Design review of the part built by this model. Coordinates are the model's own, in mm. A direction names the side the tool comes from. Coordinates: 2 decimals unless noted, no trailing zeros. Loops run counter-clockwise (first coordinate to the right, second up) from the corner with the lowest first, then second, coordinate; pieces in that order, holes last.
Q1. Add section D-D on x = 88.5. Give the boundary of the cut face in (y, z).
Q2. Draft analysis for pull direction Z (two halves, no side actions). For faces 1 (the face through (61, 51.9, 149.3)), 2 (the face through (60, 50, 0)), 3 (the face through (42.73, 51.78, 67.63)), 4 (the face through (0, 22, 54)), state which applies: released by +Z, released by -Z, zero draft, split by the parting line, or undercut.
Q3. Machinability: for faces 5 (the face through (-3.13, 4.51, 105.72)), 6 (the face through (81.41, 51.87, 74.04)), which of the approach directions +Z, -Z, +X, -X, +Y, -Y give a long, thin tool a straight path to every point of the face, cutting with its end or side? Answer none if there is none.
Q4. Add section A-A on z = 36.5. Give the boundary of the cut face in (x, y), and give its area (3 significant figures).
Q5. For P1, Ø3, axis at x = 60.5, y = 50.5, coming from the +Z side; P2, Ø3, axis at y = 52.5, z = 41.5, coming from the +X side; P3, Ø7, axis at y = 51, z = 54.5, coming from the +X side; P4, Ø1.1, axis at x = 47, y = 51, coming from the -Z side, all flat-tipped, find the tip position at first contact; note any pin that passes through.
Q6. Add section C-C on y = 21. Give the boundary of the cut face in (x, z).
Q7. Wall thickness on probe 1 along X at (y, z) = (24.5, 41); probe 2 along Y at (x, z) = (69.5, 23.5); probe 3 along X at (y, z) = (51, 26): over which ranges is each line inside the solid? List them lowest first.
Q8. Add section B-B on y = 43.5. Give the boundary of the cut face in (x, z).
```python
from build123d import *

# Parameters (mm, degrees)
BRIDA_BASE1_DEPTH          = 110
PESTA_A1_DEPTH             = 6.35
CORTAR_EXTRUIR1_REACH      = 205.181
REDONDEO1_R                = 15
CORTAR_EXTRUIR3_DEPTH      = 204.181381454
CORTAR_EXTRUIR3_DEPTH_BACK = 204.181381454
CROQUIS11_R                = 5.125
REDONDEO2_R                = 2
REDONDEO3_R                = 5


# Sheet-metal steps are written as plain solids
with BuildPart() as part:
    # Croquis1 → Brida base1 (new body)
    with BuildSketch(Plane.XY):
        with BuildLine():
            Line((0, 0), (0, 45.47))
            ThreePointArc((0, 45.47), (0.931400436, 47.718599564), (3.18, 48.65))
            Line((3.18, 48.65), (116.82, 48.65))
            ThreePointArc((116.82, 48.65), (119.068599564, 47.718599564), (120, 45.47))
            Line((120, 45.47), (120, 0))
            Line((120, 0), (126.35, 0))
            Line((126.35, 0), (126.35, 45.47))
            ThreePointArc((126.35, 45.47), (123.558727625, 52.208727625), (116.82, 55))
            Line((116.82, 55), (3.18, 55))
            ThreePointArc((3.18, 55), (-3.558727625, 52.208727625), (-6.35, 45.47))
            Line((-6.35, 45.47), (-6.35, 0))
            Line((-6.35, 0), (0, 0))
        make_face()
    extrude(amount=BRIDA_BASE1_DEPTH)

    # Croquis6 → Pestaña1 (add)
    with BuildSketch(Plane(origin=(0, 55, 0), x_dir=(1, 0, 0), z_dir=(0, 1, 0))):
        with BuildLine():
            Line((3.18, -110), (116.82, -110))
            ThreePointArc((116.82, -110), (60, -149.309581975), (3.18, -110))
        make_face()
    extrude(amount=-PESTA_A1_DEPTH)

    # Croquis9 → Cortar-Extruir1 (cut, up to next)
    with BuildSketch(Plane(origin=(0, 55, 0), x_dir=(1, 0, 0), z_dir=(0, 1, 0)), mode=Mode.PRIVATE) as cortar_extruir1_sk1:
        with BuildLine():
            Line((53.25, -115), (85.45, -115))
            Line((85.45, -115), (85.45, -93))
            ThreePointArc((85.45, -93), (79.1, -86.65), (72.75, -93))
            Line((72.75, -93), (66.75, -101))
            Line((66.75, -101), (66.75, -78))
            Line((66.75, -78), (77.45, -78))
            Line((77.45, -78), (85.45, -70))
            Line((85.45, -70), (85.45, -58))
            ThreePointArc((85.45, -58), (79.1, -51.65), (72.75, -58))
            Line((72.75, -58), (66.75, -66))
            Line((66.75, -66), (66.75, -25))
            Line((66.75, -25), (53.25, -25))
            Line((53.25, -25), (53.25, -56))
            Line((53.25, -56), (47.25, -48))
            ThreePointArc((47.25, -48), (40.9, -41.65), (34.55, -48))
            Line((34.55, -48), (34.55, -60))
            Line((34.55, -60), (42.55, -68))
            Line((42.55, -68), (53.25, -68))
            Line((53.25, -68), (53.25, -91))
            Line((53.25, -91), (47.25, -83))
            ThreePointArc((47.25, -83), (40.9, -76.65), (34.55, -83))
            Line((34.55, -83), (34.55, -105))
            Line((34.55, -105), (53.25, -105))
            Line((53.25, -105), (53.25, -115))
        make_face()
    cortar_extruir1_tool1 = extrude(cortar_extruir1_sk1.sketch, amount=-CORTAR_EXTRUIR1_REACH, mode=Mode.PRIVATE) & part.part
    add(cortar_extruir1_tool1.solids().sort_by_distance((60, 55, 76.162835))[0], mode=Mode.SUBTRACT)

    # Redondeo1
    redondeo1_edges = [part.edges().sort_by_distance(p)[0] for p in [
        (-3.175, 0, 0),
        (123.175, 0, 0),
        (-3.175, 0, 110),
        (123.175, 0, 110),
    ]]
    fillet(redondeo1_edges, radius=REDONDEO1_R)

    # Croquis11 → Cortar-Extruir3 (cut, two sides: drawn at the far end of the back side and taken through both)
    with BuildSketch(Plane.ZY.offset(-120).offset(-CORTAR_EXTRUIR3_DEPTH_BACK)):
        with Locations((20.003172622, 22.868986368)):
            Circle(CROQUIS11_R)
        with Locations((90.003172622, 22.868986368)):
            Circle(CROQUIS11_R)
    extrude(amount=CORTAR_EXTRUIR3_DEPTH + CORTAR_EXTRUIR3_DEPTH_BACK, mode=Mode.SUBTRACT)

    # Redondeo2
    redondeo2_edges = [part.edges().sort_by_distance(p)[0] for p in [
        (53.25, 51.825, 56),
        (53.25, 51.825, 25),
        (66.75, 51.825, 25),
        (66.75, 51.825, 66),
        (66.75, 51.825, 101),
        (53.25, 51.825, 91),
    ]]
    fillet(redondeo2_edges, radius=REDONDEO2_R)

    # Redondeo3
    redondeo3_edges = [part.edges().sort_by_distance(p)[0] for p in [
        (34.55, 51.825, 60),
        (47.25, 51.825, 48),
        (72.75, 51.825, 58),
        (85.45, 51.825, 70),
        (77.45, 51.825, 78),
        (66.75, 51.825, 78),
        (72.75, 51.825, 93),
        (85.45, 51.825, 115),
        (53.25, 51.825, 115),
        (53.25, 51.825, 105),
        (34.55, 51.825, 105),
        (47.25, 51.825, 83),
        (53.25, 51.825, 68),
        (42.55, 51.825, 68),
    ]]
    fillet(redondeo3_edges, radius=REDONDEO3_R - 0.0001)  # a hair under: the kernel refuses the full size


solid = part.part
```
Entries:
1. outline: (48.65, 0) - (55, 0) - (55, 142.21) - (48.65, 142.21) - close
2. face 1: released by +Z
2. face 2: released by -Z
2. face 3: undercut
2. face 4: zero draft
3. face 5: +Z, +X, -X, -Y
3. face 6: +Y, -Y
4. outline: (-6.35, 0) - (0, 0) - (0, 45.47) arc R3.18 cw to (3.18, 48.65) - (53.25, 48.65) - (53.25, 55) - (3.18, 55) arc R9.53 ccw to (-6.35, 45.47) - close; (66.75, 48.65) - (116.82, 48.65) arc R3.18 cw to (120, 45.47) - (120, 0) - (126.35, 0) - (126.35, 45.47) arc R9.53 ccw to (116.82, 55) - (66.75, 55) - close
4. area: 1,340 mm2
5. P1: stops at z = 149.31
5. P2: stops at x = 124.58
5. P3: stops at x = 126.13
5. P4: stops at z = 0
6. outline: (-6.35, 0) - (0, 0) - (0, 15.23) - (-6.35, 15.23) - close; (-6.35, 24.78) - (0, 24.78) - (0, 85.23) - (-6.35, 85.23) - close; (-6.35, 94.78) - (0, 94.78) - (0, 110) - (-6.35, 110) - close; (120, 0) - (126.35, 0) - (126.35, 15.23) - (120, 15.23) - close; (120, 24.78) - (126.35, 24.78) - (126.35, 85.23) - (120, 85.23) - close; (120, 94.78) - (126.35, 94.78) - (126.35, 110) - (120, 110) - close
7. probe 1: x = -6.35 to 0, 120 to 126.35
7. probe 2: y = 48.65 to 55
7. probe 3: x = -4.58 to 53.52, 66.48 to 124.58
8. outline: (-6.35, 0) - (0, 0) - (0, 110) - (-6.35, 110) - close; (120, 0) - (126.35, 0) - (126.35, 110) - (120, 110) - close
